Verification items for the finished model (mm, model axes). Face numbers are marked on the shaded views. Give positions to 0.01 mm unless a question says otherwise; leave off trailing zeros. Write each loop counter-clockwise with the first axis right and the second up, starting at its lowest first coordinate (ties: lowest second). Pieces come first, ordered by that corner, then holes. Notation, with made-up numbers: M -24.75,-34.5 L 13.25,-34.5 A26 cw 13.25,-20.5 Z; hole C 72,29 d8. An arc over 180 degrees is marked long. Write item = value, one per line.
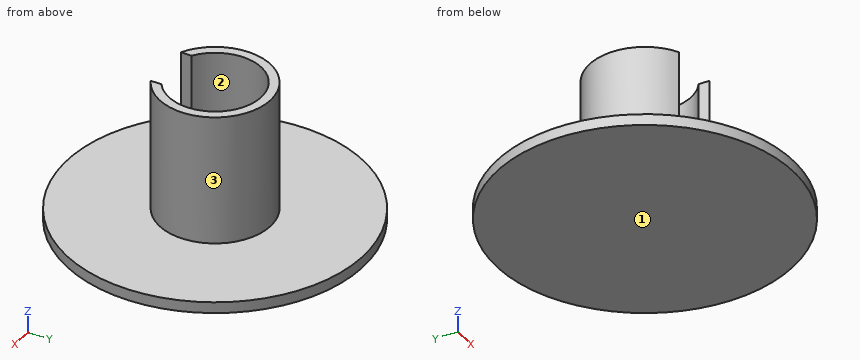
from build123d import *

# Parameters (mm, degrees)
F0_R     = 40
F1_DEPTH = 3
F2_R     = 15
F2_R_2   = 12.5
F3_DEPTH = 35
F4_W     = 14
F4_H     = 50
F5_DEPTH = 35


with BuildPart() as f1:
    # F0 (on Top) → F1 (new body)
    with BuildSketch(Plane.XY):
        Circle(F0_R)
    extrude(amount=F1_DEPTH)

    # F2 (on face) → F3 (join)
    with BuildSketch(Plane.XY.offset(3)):
        Circle(F2_R)
        Circle(F2_R_2, mode=Mode.SUBTRACT)
    extrude(amount=F3_DEPTH)

    # F4 (on face) → F5 (cut)
    with BuildSketch(Plane.XY.offset(38)):
        with Locations((0, -25)):
            Rectangle(F4_W, F4_H)
    extrude(amount=-F5_DEPTH, mode=Mode.SUBTRACT)


solid = f1.part
1) Draft check along X on the marked faces 1, 2 and 3. Enter one of: +X half, -X half, draft (parallel to the pull), parting line (faces both ways), or undercut.
From the geometry:
face_1 = draft
face_2 = undercut
face_3 = parting line
2) Material ranges on probe 1 along X at (y, z) = (0, 18.5); probe 2 along Z at (x, y) = (-24.5, -15.5); probe 3 along X at (y, z) = (-7.5, 14), recorded low to high. Write a range as from..to.
From the geometry:
probe_1 = -15..-12.5, 12.5..15
probe_2 = 0..3
probe_3 = -12.99..-10, 10..12.99
3) Cross-section at B-B on y = 0. Record the boundary of the cut face in (x, z), plus the area to 3 significant figures.
From the geometry:
outline = M -40,0 L 40,0 L 40,3 L 15,3 L 15,38 L 12.5,38 L 12.5,3 L -12.5,3 L -12.5,38 L -15,38 L -15,3 L -40,3 Z
area = 415 mm^2
4) Cross-section at D-D on x = 14. Record the boundary of the cut face in (y, z), plus the area to 3 significant figures.
From the geometry:
outline = M -37.47,0 L 37.47,0 L 37.47,3 L 5.39,3 L 5.39,38 L -5.39,38 L -5.39,3 L -37.47,3 Z
area = 602 mm^2
5) Cross-section at C-C on z = 14.5. Record the boundary of the cut face in (x, y), plus the area to 3 significant figures.
From the geometry:
outline = M -7,-13.27 L -7,-10.36 A12.5 cw long 7,-10.36 L 7,-13.27 A15 ccw long Z
area = 179 mm^2
6) Depth check by flat-ended pin: P1, Ø2, axis at y = -4.5, z = 33.5, coming from the +X side; P2, Ø5, axis at x = -11, y = 16.5, coming from the +Z side; P3, Ø10, axis at x = 14, z = 7.5, coming from the -Y side. Enter the tip coordinate at first touch or a pass-through.
From the geometry:
P1 = 14.59
P2 = 3
P3 = -38.21
7) Cross-section at A-A on x = 0. Record the boundary of the cut face in (y, z), plus the area to 4 significant figures.
From the geometry:
outline = M -40,0 L 40,0 L 40,3 L 15,3 L 15,38 L 12.5,38 L 12.5,3 L -40,3 Z
area = 327.5 mm^2
